from build123d import *

# Parameters (mm, degrees)
SKETCH1_R             = 20
BOSS_EXTRUDE1_DEPTH   = 4
CUT_EXTRUDE1_DEPTH    = 3
M4X0_7_TAPPED_HOLE1_D = 3.3
SKETCH5_R             = 4.9
CUT_EXTRUDE2_DEPTH    = 5
SKETCH6_R             = 8
CUT_EXTRUDE3_DEPTH    = 3


with BuildPart() as part:
    # Sketch1 → Boss-Extrude1 (new body)
    with BuildSketch(Plane.XY):
        Circle(SKETCH1_R)
    extrude(amount=BOSS_EXTRUDE1_DEPTH)

    # Sketch2 → Cut-Extrude1 (cut)
    with BuildSketch(Plane.XY.offset(4)):
        with BuildLine():
            Line((-3, 17.8), (-3, 25))
            Line((-3, 25), (3, 25))
            Line((3, 25), (3, 17.8))
            ThreePointArc((3, 17.8), (0, 14.8), (-3, 17.8))
        make_face()
        with BuildLine():
            Line((16.915252187, -6.301923789), (23.150635095, -9.901923789))
            Line((23.150635095, -9.901923789), (20.150635095, -15.098076211))
            Line((20.150635095, -15.098076211), (13.915252187, -11.498076211))
            ThreePointArc((13.915252187, -11.498076211), (12.817175976, -7.4), (16.915252187, -6.301923789))
        make_face()
        with BuildLine():
            Line((-13.915252187, -11.498076211), (-20.150635095, -15.098076211))
            Line((-20.150635095, -15.098076211), (-23.150635095, -9.901923789))
            Line((-23.150635095, -9.901923789), (-16.915252187, -6.301923789))
            ThreePointArc((-16.915252187, -6.301923789), (-12.817175976, -7.4), (-13.915252187, -11.498076211))
        make_face()
    extrude(amount=-CUT_EXTRUDE1_DEPTH, mode=Mode.SUBTRACT)

    # M4x0.7 Tapped Hole1 (through all)
    with Locations(Plane.XY.offset(4)):
        with Locations((-8.838834765, 8.838834765), (8.838834765, 8.838834765), (8.838834765, -8.838834765), (-8.838834765, -8.838834765)):
            Hole(M4X0_7_TAPPED_HOLE1_D / 2)

    # Sketch5 → Cut-Extrude2 (cut, through all)
    with BuildSketch(Plane.XY.offset(4)):
        Circle(SKETCH5_R)
    extrude(amount=-CUT_EXTRUDE2_DEPTH, mode=Mode.SUBTRACT)

    # Sketch6 → Cut-Extrude3 (cut)
    with BuildSketch(Plane(origin=(0, 0, 0), x_dir=(-1, 0, 0), z_dir=(0, 0, -1))):
        Circle(SKETCH6_R)
    extrude(amount=-CUT_EXTRUDE3_DEPTH, mode=Mode.SUBTRACT)


solid = part.part
Build history of the part. All positions in model axes, mm. A direction names the side the tool comes from. Give positions to 0.01 mm unless a question says otherwise; leave off trailing zeros. Write each loop counter-clockwise with the first axis right and the second up, starting at its lowest first coordinate (ties: lowest second). Pieces come first, ordered by that corner, then holes. Notation, with made-up numbers: (16.25, 60) - (49.25, 60) arc R18 ccw to (49.25, 82) - close; hole circle Ø10 at (35, 78.25). An arc over 180 degrees is marked (long way). Use one line per item in the form item = value. Start each with the question number.
1. Drop flat-ended pins along their axis: pin 1 Ø2.5 at (x, y) = (-1, 17) entering from +Z; pin 2 Ø17.5 at (x, y) = (0.5, -0.5) entering from -Z; pin 3 Ø1.6 at (y, z) = (19, 2) entering from -X; pin 4 Ø0.6 at (y, z) = (18.5, 2) entering from +X. Give the stop position or say it passes through.
2. Band-saw the part on B-B on y = 10. Write the cut outline in (x, z), plus the area to 3 significant figures.
3. Band-saw the part on A-A on x = 0. Write the cut outline in (y, z).
4. Probe line 1 (X direction, y = -9, z = 3.4); line 2 (X direction, y = 9, z = 2); line 3 (Y direction, x = 0, z = 3.3). List the from-to ranges inside material, lowest first. Write a range as [from, to].
5. Band-saw the part on D-D on z = 1.65. Write the cut outline in (x, y).
6. Two-plate mould, pull along Y, no slides. Class faces 1 (the face through (0.1, 14.8, 2.5)), 2 (the face through (10.487, -8.766, 1.972)), 3 (the face through (3, 19, 3)): released by +Y, released by -Y, zero draft, split by the parting line, or undercut.
7. 3-axis set-ups, long thin cutter, end or side, ignore diameter. For faces 4 (the face through (1.73, -7.81, 1.48)), 5 (the face through (-12.851, -7.343, 2.521)), 6 (the face through (-3, 19, 3)), 7 (the face through (17.76, -6.79, 2.52)), 8 (the face through (14.782, -11.998, 2.521)): which of +Z, -Z, +X, -X, +Y, -Y reach the whole face in a straight line?
Conclusion:
q1.pin_1 = 1
q1.pin_2 = 0
q1.pin_3 = -8.29
q1.pin_4 = 8.29
q2.outline = (-17.32, 0) - (-10.01, 0) - (-10.01, 4) - (-17.32, 4) - close; (-7.67, 0) - (7.67, 0) - (7.67, 4) - (-7.67, 4) - close; (10.01, 0) - (17.32, 0) - (17.32, 4) - (10.01, 4) - close
q2.area = 120 mm²
q3.outline = (-20, 0) - (-8, 0) - (-8, 3) - (-4.9, 3) - (-4.9, 4) - (-20, 4) - close; (4.9, 3) - (8, 3) - (8, 0) - (20, 0) - (20, 1) - (14.8, 1) - (14.8, 4) - (4.9, 4) - close
q4.line_1 = [-12.42, -10.48], [-7.2, 7.2], [10.48, 12.42]
q4.line_2 = [-17.86, -10.48], [-7.2, 7.2], [10.48, 17.86]
q4.line_3 = [-20, -4.9], [4.9, 14.8]
q5.outline = (-18.62, -7.29) - (-16.92, -6.3) arc R3 cw to (-13.92, -11.5) - (-15.62, -12.48) arc R20 ccw to (15.62, -12.48) - (13.92, -11.5) arc R3 cw to (16.92, -6.3) - (18.62, -7.29) arc R20 ccw to (3, 19.77) - (3, 17.8) arc R3 cw to (-3, 17.8) - (-3, 19.77) arc R20 ccw to start; hole circle Ø3.3 at (-8.84, -8.84); hole circle Ø3.3 at (-8.84, 8.84); hole circle Ø16 at (0, 0); hole circle Ø3.3 at (8.84, -8.84); hole circle Ø3.3 at (8.84, 8.84)
q6.face_1 = released by +Y
q6.face_2 = undercut
q6.face_3 = zero draft
q7.face_4 = -Z
q7.face_5 = +Z
q7.face_6 = +Z, +Y
q7.face_7 = +Z, -Y
q7.face_8 = +Z, +X
